Read the model definition and answer for the solid it produces. Units are mm, in the model's axes. A direction names the side the tool comes from. Coordinates: 2 decimals unless noted, no trailing zeros. Write each loop counter-clockwise with the first axis right and the second up, starting at its lowest first coordinate (ties: lowest second). Pieces come first, ordered by that corner, then holes. Notation, with made-up numbers: (68.25, 31) - (95.25, 31) arc R32 cw to (95.25, 61) - close; hole circle Ø3 at (88.5, -18.75). An arc over 180 degrees is marked (long way). Use a Markdown table: item, result.
from build123d import *

# Parameters (mm, degrees)
F6_DEPTH  = 381
F6_TAPER  = 5
F7_DEPTH  = 381
F4_W      = 498.475
F4_H      = 203.2
F8_DEPTH  = 336.55
F9_R      = 50.8
F10_R     = 50.8
F11_R     = 25.4
F5_W      = 762
F5_H      = 1231.9
F12_DEPTH = 6.35


with BuildPart() as f6:
    # F2 (on offset) → F6 (new body, through all)
    with BuildSketch(Plane.XY.offset(381)):
        with BuildLine():
            add(Edge.make_bspline(
                [(0, 228.6), (-307.9586335857, 228.6), (-153.9793167929, -114.3), (0, -457.2), (153.9793167929, -114.3), (307.9586335857, 228.6), (0, 228.6)],
                knots=[0, 0, 0, 2.0943951024, 2.0943951024, 4.1887902048, 4.1887902048, 6.2831853072, 6.2831853072, 6.2831853072], degree=2, weights=[1, 0.5, 1, 0.5, 1, 0.5, 1]))
        make_face()
    extrude(amount=-F6_DEPTH, taper=F6_TAPER)

    # F3 (on Top) → F7 (join, through all)
    with BuildSketch(Plane.XY):
        Polygon((-101.6, 469.9), (-101.6, 0), (0, 0), (101.6, 0), (101.6, 469.9), align=None)
    extrude(amount=F7_DEPTH)

    # F4 (on offset) → F8 (join, through all)
    with BuildSketch(Plane.XY.offset(381)):
        with Locations((0, 368.3)):
            Rectangle(F4_W, F4_H)
    extrude(amount=F8_DEPTH)

    # F9
    f9_edges = [f6.edges().sort_by_distance(p)[0] for p in [
        (-101.6, 469.9, 190.5),
        (101.6, 469.9, 190.5),
    ]]
    fillet(f9_edges, radius=F9_R)

    # F10
    f10_edges = [f6.edges().sort_by_distance(p)[0] for p in [
        (101.6, 164.265069, 190.329553),
        (-101.6, 164.265069, 190.329553),
    ]]
    fillet(f10_edges, radius=F10_R)

    # F11
    f11_edges = [f6.edges().sort_by_distance(p)[0] for p in [
        (249.2375, 266.7, 549.275),
        (249.2375, 469.9, 549.275),
        (-249.2375, 266.7, 549.275),
        (-249.2375, 469.9, 549.275),
    ]]
    fillet(f11_edges, radius=F11_R)

    # F5 (on Top) → F12 (join)
    with BuildSketch(Plane.XY):
        with Locations((0, -146.05)):
            Rectangle(F5_W, F5_H)
    extrude(amount=F12_DEPTH)


solid = f6.part
(1) Each of these flat-tipped pins is pushed along its axis until it touches: P1, Ø1, axis at x = -64.5, z = 111, coming from the -Y side; P2, Ø10, axis at x = 193, y = 220.5, coming from the +Z side; P3, Ø3, axis at x = 105.5, y = -514, coming from the +Z side. Where does it stop, or does it pass through?
Report:
| item | result |
|---|---|
| P1 | stops at y = -186.32 |
| P2 | stops at z = 6.35 |
| P3 | stops at z = 6.35 |
(2) A cutting plane is placed at B-B, the plane x = -288.5. Write down the section's boundary in (y, z), and give its area (3 significant figures).
Report:
| item | result |
|---|---|
| outline | (-762, 0) - (469.9, 0) - (469.9, 6.35) - (-762, 6.35) - close |
| area | 7,820 mm² |
(3) A cutting plane is placed at A-A, the plane z = 667.5. Write down the section's boundary in (x, y).
Report:
| item | result |
|---|---|
| outline | (-249.24, 292.1) arc R25.4 ccw to (-223.84, 266.7) - (223.84, 266.7) arc R25.4 ccw to (249.24, 292.1) - (249.24, 444.5) arc R25.4 ccw to (223.84, 469.9) - (-223.84, 469.9) arc R25.4 ccw to (-249.24, 444.5) - close |
(4) Straight lines are drawn through the part: L1, parallel to Z at x = 171.5, y = -194; L2, parallel to Y at x = -118.5, z = 384. For each, find the intervals that lie inside material, in ascending order.
Report:
| item | result |
|---|---|
| L1 | z = 0 to 6.35 |
| L2 | y = 266.7 to 469.9 |
(5) The mould has two halves that part along Z. Classify faces 5 (the flat face through (-3, 370, 717.55)), 6 (the cylindrical face through (86.324, 455.414, 196.298)), 7 (the cylindrical face through (-241.599, 273.943, 551.631)): pulls with the +Z half, pulls with the -Z half, needs draft (parallel to the pull), parting line crosses it, or undercut.
Report:
| item | result |
|---|---|
| face 5 | pulls with the +Z half |
| face 6 | undercut |
| face 7 | needs draft |
(6) A cutting plane is placed at C-C, the plane y = -674.5. Write down the section's boundary in (x, z).
Report:
| item | result |
|---|---|
| outline | (-381, 0) - (381, 0) - (381, 6.35) - (-381, 6.35) - close |
(7) For faces 1 (the cylindrical face through (-86.324, 455.414, 196.298)), 2 (the flat face through (-2, 23, 381)), 3 (the cylindrical face through (241.599, 462.657, 551.631)), 4 (the flat face through (171, 370, 381)), determine the directions among +Z, -Z, +X, -X, +Y, -Y from which every point of the face is accessible in a straight line to the end or side of a thin tool.
Report:
| item | result |
|---|---|
| face 1 | -X, +Y |
| face 2 | +Z, +X, -X, -Y |
| face 3 | +Z, +X, +Y |
| face 4 | +X, +Y |
